Read the model definition and answer for the solid it produces. Units are mm, in the model's axes. A direction names the side the tool comes from. Coordinates: 2 decimals unless noted, no trailing zeros. Order: outer loops, then holes, each group sorted by start corner. A loop starts at its lowest first (then second) coordinate and runs counter-clockwise, first axis right, second up. Notation, with made-up numbers: (-28, -9.75) -> (21, -9.75) arc R17 cw to (21, 21.25) -> close; hole circle Ø8 at (74.25, 64.25). An arc over 180 degrees is marked (long way). Answer in a Markdown table with one row per item.
from build123d import *

# Parameters (mm, degrees)
F0_W     = 500
F0_H     = 30
F0_W_2   = 30
F0_H_2   = 800
F1_DEPTH = 50
F2_DEPTH = 700


with BuildPart() as f1:
    # F0 (on Top) → F1 (new body)
    with BuildSketch(Plane.XY):
        Polygon((-530.000132, 0), (-500, 0), (-500, 800), (-529.910707, 800), align=None)
        Polygon((-529.910707, 800), (-500, 800), (-500, 830), (-529.999868, 830), align=None)
        with Locations((-250, 815)):
            Rectangle(F0_W, F0_H)
        with Locations((15, 815)):
            Rectangle(F0_W_2, F0_H)
        with Locations((15, 400)):
            Rectangle(F0_W_2, F0_H_2)
        with Locations((15, -15)):
            Rectangle(F0_W_2, F0_H)
        Polygon((0, -30), (0, 0), (-500, 0), (-499.91084, -29.999868), align=None)
        Polygon((-499.91084, -29.999868), (-500, 0), (-530.000132, 0), (-529.910707, -30.089028), align=None)
    extrude(amount=-F1_DEPTH)

    # F0 (on Top) → F2 (join)
    with BuildSketch(Plane.XY):
        with Locations((15, -15)):
            Rectangle(F0_W_2, F0_H)
        Polygon((-499.91084, -29.999868), (-500, 0), (-530.000132, 0), (-529.910707, -30.089028), align=None)
        Polygon((-529.910707, 800), (-500, 800), (-500, 830), (-529.999868, 830), align=None)
        with Locations((15, 815)):
            Rectangle(F0_W_2, F0_H)
    extrude(amount=-F2_DEPTH)


solid = f1.part
Q1. The part is cut by section B-B (x = -22). Write down the section's boundary in (y, z), then the cut area to 3 significant figures.
Outcome:
| item | result |
|---|---|
| outline | (-30, -50) -> (0, -50) -> (0, 0) -> (-30, 0) -> close; (800, -50) -> (830, -50) -> (830, 0) -> (800, 0) -> close |
| area | 3,000 mm² |
Q2. Given pin 1 (9 mm diameter, centred on x = 12.5, z = -359.5, fed in from -Y); pin 2 (9 mm diameter, centred on y = -17, z = -424.5, fed in from -X); pin 3 (9 mm diameter, centred on x = -509.5, y = 417, fed in from -Z), each flat-ended and moving along its own axis, determine where each tip first touches the part or whether it passes through.
Outcome:
| item | result |
|---|---|
| pin 1 | y = -30 |
| pin 2 | x = -529.96 |
| pin 3 | z = -50 |
Q3. For faces 4 (the face through (-515, 406, -50)), 5 (the face through (0, 406, -25)), 6 (the face through (-254, 815, -50)), 7 (the face through (-500.2, 402, 0)), determine the directions among +Z, -Z, +X, -X, +Y, -Y from which every point of the face is accessible in a straight line to the end or side of a thin tool.
Outcome:
| item | result |
|---|---|
| face 4 | -Z, +X, -X |
| face 5 | +Z, -Z |
| face 6 | -Z, +Y, -Y |
| face 7 | +Z, +X, -X, +Y, -Y |
Q4. The part is cut by section A-A (z = -75). Write down the section's boundary in (x, y).
Outcome:
| item | result |
|---|---|
| outline | (-530, 0) -> (-529.91, -30.09) -> (-499.91, -30) -> (-500, 0) -> close; (-530, 830) -> (-529.91, 800) -> (-500, 800) -> (-500, 830) -> close; (0, -30) -> (30, -30) -> (30, 0) -> (0, 0) -> close; (0, 800) -> (30, 800) -> (30, 830) -> (0, 830) -> close |
Q5. Consider line 1 (Y direction, x = -505, z = -659) (3 decimals). Determine where the line is inside the solid, lowest interval first.
Outcome:
| item | result |
|---|---|
| line 1 | -30.015 to 0, 800 to 830 |
Q6. For a pull along X with two mould halves and no side action, classify faces 1 (the face through (-515, 815, -700)), 2 (the face through (0, -15, -370)), 3 (the face through (-247, 0, -25)) as pulls with the +X half, pulls with the -X half, needs draft (parallel to the pull), parting line crosses it, or undercut.
Outcome:
| item | result |
|---|---|
| face 1 | needs draft |
| face 2 | undercut |
| face 3 | undercut |
Q7. The part is cut by section C-C (y = 218.5). Write down the section's boundary in (x, z), then the cut area to 3 significant figures.
Outcome:
| item | result |
|---|---|
| outline | (-529.98, -50) -> (-500, -50) -> (-500, 0) -> (-529.98, 0) -> close; (0, -50) -> (30, -50) -> (30, 0) -> (0, 0) -> close |
| area | 3,000 mm² |
